```python
from build123d import *

# Parameters (mm, degrees)
SKETCH1_R           = 2.5
BOSS_EXTRUDE1_DEPTH = 1
SKETCH1_3_W         = 3.81
SKETCH1_3_H         = 5
BOSS_EXTRUDE2_DEPTH = 10.16
BOSS_EXTRUDE3_DEPTH = 6
BOSS_EXTRUDE4_DEPTH = 5
FILLET2_R           = 2
CHAMFER1_SIZE       = 0.6
FILLET3_R           = 0.6


with BuildPart() as part:
    # Sketch1 → Boss-Extrude1 (new body)
    with BuildSketch(Plane(origin=(0, 0, 0), x_dir=(1, 0, 0), z_dir=(0, 1, 0))):
        Polygon((-3.81, 0), (-5.56, 0), (-5.56, -1.6), (86.16, -1.6), (86.16, 0), (84.41, 0), (84.41, 20.6), (86.16, 20.6), (86.16, 22.2), (-5.56, 22.2), (-5.56, 20.6), (-3.81, 20.6), align=None)
        with Locations((20.15, 10.3)):
            Circle(SKETCH1_R, mode=Mode.SUBTRACT)
        with Locations((60.45, 10.3)):
            Circle(SKETCH1_R, mode=Mode.SUBTRACT)
    extrude(amount=-BOSS_EXTRUDE1_DEPTH)

    # Sketch1<3> → Boss-Extrude2 (add)
    with BuildSketch(Plane(origin=(0, 0, 0), x_dir=(1, 0, 0), z_dir=(0, 1, 0))):
        with Locations((-1.905, 10.3)):
            Rectangle(SKETCH1_3_W, SKETCH1_3_H)
        with Locations((82.505, 10.3)):
            Rectangle(SKETCH1_3_W, SKETCH1_3_H)
    extrude(amount=BOSS_EXTRUDE2_DEPTH)

    # Sketch1<4> → Boss-Extrude3 (add)
    with BuildSketch(Plane(origin=(0, 0, 0), x_dir=(1, 0, 0), z_dir=(0, 1, 0))):
        Polygon((80.6, 0), (0, 0), (-3.81, 0), (-5.56, 0), (-5.56, -1.6), (86.16, -1.6), (86.16, 0), (84.41, 0), align=None)
        Polygon((-3.81, 20.6), (0, 20.6), (80.6, 20.6), (84.41, 20.6), (86.16, 20.6), (86.16, 22.2), (-5.56, 22.2), (-5.56, 20.6), align=None)
    extrude(amount=BOSS_EXTRUDE3_DEPTH)

    # Sketch2 → Boss-Extrude4 (add)
    with BuildSketch(Plane.XY.offset(-7.8)):
        Polygon((0, 10.16), (1.927427041, 8.905), (0, 7.16), align=None)
    boss_extrude4 = extrude(amount=-BOSS_EXTRUDE4_DEPTH)

    # Mirror1: Boss-Extrude4 across plane
    add(boss_extrude4.mirror(Plane(origin=(40.3, 0, 0), x_dir=(0, 0, 1), z_dir=(1, 0, 0))))

    # Fillet2
    fillet2_edges = [part.edges().sort_by_distance(p)[0] for p in [
        (0, 0, -10.3),
        (-1.905, 0, -12.8),
        (-1.905, 0, -7.8),
        (82.505, 0, -7.8),
        (80.6, 0, -10.3),
        (82.505, 0, -12.8),
    ]]
    fillet(fillet2_edges, radius=FILLET2_R)

    # Chamfer1
    chamfer1_edges = [part.edges().sort_by_distance(p)[0] for p in [
        (17.65, 0, -10.3),
        (57.95, 0, -10.3),
    ]]
    chamfer(chamfer1_edges, length=CHAMFER1_SIZE)

    # Fillet3
    fillet3_edges = [part.edges().sort_by_distance(p)[0] for p in [
        (-5.56, 2.5, -20.6),
        (-5.56, 2.5, -22.2),
        (86.16, 2.5, -22.2),
        (86.16, 2.5, -20.6),
        (86.16, 2.5, 0),
        (86.16, 2.5, 1.6),
        (-5.56, 2.5, 1.6),
        (-5.56, 2.5, 0),
    ]]
    fillet(fillet3_edges, radius=FILLET3_R)


solid = part.part
```
Input: part model. Units: mm. Frame: model coordinates. A direction names the side the tool comes from. Round coordinates to 2 decimals unless told otherwise and drop trailing zeros. Order: outer loops, then holes, each group sorted by start corner. A loop starts at its lowest first (then second) coordinate and runs counter-clockwise, first axis right, second up. Notation, with made-up numbers: (76, 17) - (82, 17) arc R32 ccw to (82, 52) - close; hole circle Ø7 at (-10, 87.25). An arc over 180 degrees is marked (long way). One line per question, with ' | ' between items. Start each with the question number.
1) Set-up query: faces 1 (the flat face through (79.65, 9.54, -10.26)), 2 (the flat face through (82, 6, -12.8)), 3 (the flat face through (84.41, 3, -10)), 4 (the flat face through (40, 0, -10)). Return all of +Z, -Z, +X, -X, +Y, -Y with unobstructed straight access to the full face (end or side cutting, diameter ignored); none if empty.
2) Pull-direction query (Z, two-part tool) for faces 5 (the flat face through (41, 2, 0)), 6 (the flat face through (40, -1, -10)), 7 (the flat face through (40, 2, 1.6)); classes: +Z half, -Z half, draft (parallel to the pull), parting line (faces both ways), or undercut.
3) Ray query, probe 1 along X at (y, z) = (-0.8, -10.3); probe 2 along Z at (x, y) = (20.15, -0.75); probe 3 along Z at (x, y) = (38, 3.75). Return the intervals inside material, ascending.
4) Cut plane D-D, the plane x = 48. Return the cut outline in (y, z), then the cut area to 3 significant figures.
5) Cut plane C-C, the plane x = 60.45. Return the cut outline in (y, z).
6) Cut plane A-A, the plane z = -10.3. Return the cut outline in (x, y) (3 decimals).
7) Contact query for flat-ended pins moving along their axis: P1, Ø5.5, axis at y = 7.5, z = -12.5, coming from the +X side; P2, Ø12, axis at x = 26.5, z = -9, coming from the +Y side; P3, Ø5.5, axis at y = 4.5, z = -10, coming from the -X side; P4, Ø4.5, axis at x = 80.5, y = 7, coming from the -Z side. Output: stop coordinate, or through.
8) Cut plane B-B, the plane y = 4. Return the cut outline in (x, z).
Worked out:
1) face 1: +Z, -Z, +Y | face 2: +X, -X, +Y | face 3: +X, +Y, -Y | face 4: +Y
2) face 5: undercut | face 6: draft | face 7: +Z half
3) probe 1: x = -3.81 to 17.65, 22.65 to 57.95, 62.95 to 84.41 | probe 2: z = -22.2 to -12.8, -7.8 to 1.6 | probe 3: z = -22.2 to -20.6, 0 to 1.6
4) outline: (-1, -22.2) - (6, -22.2) - (6, -20.6) - (0, -20.6) - (0, 0) - (6, 0) - (6, 1.6) - (-1, 1.6) - close | area: 43.0 mm^2
5) outline: (-1, -22.2) - (6, -22.2) - (6, -20.6) - (0, -20.6) - (0, -13.4) - (-0.6, -12.8) - (-1, -12.8) - close; (-1, -7.8) - (-0.6, -7.8) - (0, -7.2) - (0, 0) - (6, 0) - (6, 1.6) - (-1, 1.6) - close
6) outline: (-3.81, -1) - (17.65, -1) - (17.65, -0.6) - (17.05, 0) - (2, 0) arc R2 cw to (0, 2) - (0, 7.16) - (1.927, 8.905) - (0, 10.16) - (-3.81, 10.16) - close; (22.65, -1) - (57.95, -1) - (57.95, -0.6) - (57.35, 0) - (23.25, 0) - (22.65, -0.6) - close; (62.95, -1) - (84.41, -1) - (84.41, 10.16) - (80.6, 10.16) - (78.673, 8.905) - (80.6, 7.16) - (80.6, 2) arc R2 cw to (78.6, 0) - (63.55, 0) - (62.95, -0.6) - close
7) P1: stops at x = 84.41 | P2: stops at y = 0 | P3: stops at x = -3.81 | P4: stops at z = -22.2
8) outline: (-5.56, -21.6) arc R0.6 ccw to (-4.96, -22.2) - (85.56, -22.2) arc R0.6 ccw to (86.16, -21.6) - (86.16, -21.2) arc R0.6 ccw to (85.56, -20.6) - (-4.96, -20.6) arc R0.6 ccw to (-5.56, -21.2) - close; (-5.56, 0.6) arc R0.6 ccw to (-4.96, 0) - (85.56, 0) arc R0.6 ccw to (86.16, 0.6) - (86.16, 1) arc R0.6 ccw to (85.56, 1.6) - (-4.96, 1.6) arc R0.6 ccw to (-5.56, 1) - close; (-3.81, -12.8) - (0, -12.8) - (0, -7.8) - (-3.81, -7.8) - close; (80.6, -12.8) - (84.41, -12.8) - (84.41, -7.8) - (80.6, -7.8) - close
